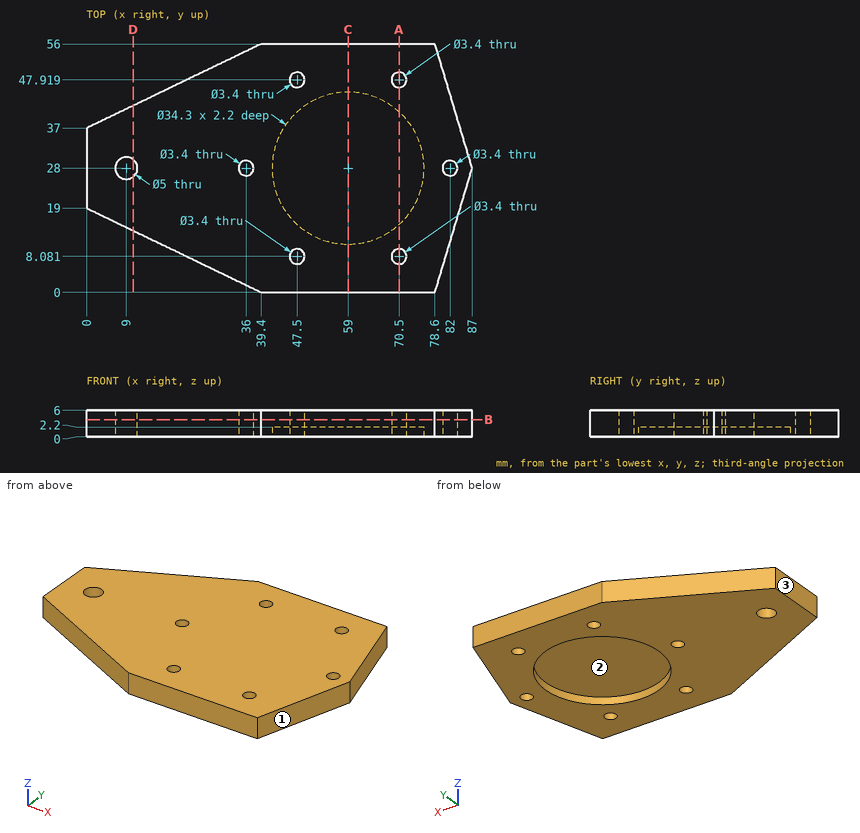
The figure shows three views and two pictorial views of one solid part (mm, origin at its lowest corner). Answer the questions. Give positions to 0.01 mm unless a question says otherwise; leave off trailing zeros. Order: outer loops, then holes, each group sorted by start corner. A loop starts at its lowest first (then second) coordinate and runs counter-clockwise, first axis right, second up. Notation, with made-up numbers: (-9.5, -22.75) -> (32.5, -22.75) arc R15 ccw to (32.5, -4.75) -> close; hole circle Ø11 at (73.5, 32.25). An arc over 180 degrees is marked (long way). Write each question's results on one line, items separated by ' | '.
Q1. The part is cut by section A-A, the plane x = 70.5. Give the vertices of the cut face in (y, z).
Checked values:
outline: (0, 0) -> (6.38, 0) -> (6.38, 6) -> (0, 6) -> close; (9.78, 0) -> (15.28, 0) -> (15.28, 2.2) -> (40.72, 2.2) -> (40.72, 0) -> (46.22, 0) -> (46.22, 6) -> (9.78, 6) -> close; (49.62, 0) -> (56, 0) -> (56, 6) -> (49.62, 6) -> close
Q2. The part is cut by section D-D, the plane x = 10.5. Give the vertices of the cut face in (y, z).
Checked values:
outline: (13.94, 0) -> (26, 0) -> (26, 6) -> (13.94, 6) -> close; (30, 0) -> (42.06, 0) -> (42.06, 6) -> (30, 6) -> close
Q3. Each of these flat-tipped pins is pushed along its axis until it touches: P1, Ø1, axis at x = 11.5, z = 3, coming from the +Y side; P2, Ø1.5, axis at x = 20.5, z = 1.5, coming from the +Y side; P3, Ø3, axis at y = 13.5, z = 2.5, coming from the +X side. Where does it stop, or does it pass through?
Checked values:
P1: stops at y = 42.79 | P2: stops at y = 47.25 | P3: stops at x = 83.1
Q4. Determine the mould class of the marked faces 1, 2 and 3 for opening direction Y: pulls with the +Y half, pulls with the -Y half, needs draft (parallel to the pull), parting line crosses it, or undercut.
Checked values:
face 1: pulls with the -Y half | face 2: undercut | face 3: needs draft
Q5. Straight lines are drawn through the part: probe 1 along Y at (x, z) = (47.5, 4.5); probe 2 along Y at (x, z) = (59, 1.25); probe 3 along Z at (x, y) = (52.5, 41). For each, find the intervals that lie inside material, in ascending order. Write a range as from..to.
Checked values:
probe 1: y = 0..6.38, 9.78..46.22, 49.62..56 | probe 2: y = 0..10.85, 45.15..56 | probe 3: z = 2.2..6
Q6. The part is cut by section C-C, the plane x = 59. Give the vertices of the cut face in (y, z).
Checked values:
outline: (0, 0) -> (10.85, 0) -> (10.85, 2.2) -> (45.15, 2.2) -> (45.15, 0) -> (56, 0) -> (56, 6) -> (0, 6) -> close
Q7. The part is cut by section B-B, the plane z = 3.9. Give the vertices of the cut face in (x, y), and give its area (3 significant figures).
Checked values:
outline: (0, 19) -> (39.4, 0) -> (78.6, 0) -> (87, 28) -> (78.6, 56) -> (39.4, 56) -> (0, 37) -> close; hole circle Ø5 at (9, 28); hole circle Ø3.4 at (36, 28); hole circle Ø3.4 at (47.5, 8.08); hole circle Ø3.4 at (47.5, 47.92); hole circle Ø3.4 at (70.5, 8.08); hole circle Ø3.4 at (70.5, 47.92); hole circle Ø3.4 at (82, 28) | area: 3,810 mm^2
